The listing builds one solid part. Answer for the finished solid, in the listing's coordinates (mm). Coordinates: 2 decimals unless noted, no trailing zeros. Order: outer loops, then holes, each group sorted by start corner. A loop starts at its lowest first (then second) coordinate and runs counter-clockwise, first axis right, second up. Notation, with made-up numbers: (77.5, 67) -> (116.5, 67) arc R24 ccw to (116.5, 96) -> close; hole circle Ø8 at (69.5, 78). An arc over 180 degrees is marked (long way). Answer in a Markdown table with one row per item.
```python
from build123d import *

# Parameters (mm, degrees)
BOSS_EXTRUDE1_DEPTH = 17
SKETCH2_R           = 2.5
CUT_EXTRUDE1_DEPTH  = 127.546434165
SKETCH3_R           = 1.7
CUT_EXTRUDE2_DEPTH  = 127.546434165


with BuildPart() as part:
    # Sketch1 → Boss-Extrude1 (new body)
    with BuildSketch(Plane.XY):
        with BuildLine():
            Line((3.328897286, -9.429657621), (-95.00665407, -44.144486432))
            ThreePointArc((-95.00665407, -44.144486432), (-113.476816743, -36.586001098), (-108.091360043, -17.369485653))
            Line((-108.091360043, -17.369485653), (-5.394240028, 48.420342898))
            ThreePointArc((-5.394240028, 48.420342898), (2.050554972, 49.787503477), (8.320502943, 45.547001962))
            Line((8.320502943, 45.547001962), (28.320502943, 15.547001962))
            ThreePointArc((28.320502943, 15.547001962), (29.664996488, 7.433320648), (24.472135955, 1.05572809))
            Line((24.472135955, 1.05572809), (4.472135955, -8.94427191))
            ThreePointArc((4.472135955, -8.94427191), (3.908059586, -9.204730863), (3.328897286, -9.429657621))
        make_face()
    extrude(amount=BOSS_EXTRUDE1_DEPTH)

    # Sketch2 → Cut-Extrude1 (cut, through all)
    with BuildSketch(Plane.XY.offset(17)):
        with Locations((-100, -30)):
            Circle(SKETCH2_R)
        Circle(SKETCH2_R)
        with Locations((0, 40)):
            Circle(SKETCH2_R)
        with Locations((20, 10)):
            Circle(SKETCH2_R)
    extrude(amount=-CUT_EXTRUDE1_DEPTH, mode=Mode.SUBTRACT)

    # Sketch3 → Cut-Extrude2 (cut, through all)
    with BuildSketch(Plane.XY.offset(17)):
        with Locations((-108.5, -30)):
            Circle(SKETCH3_R)
        with Locations((-91.5, -30)):
            Circle(SKETCH3_R)
    extrude(amount=-CUT_EXTRUDE2_DEPTH, mode=Mode.SUBTRACT)


solid = part.part
```
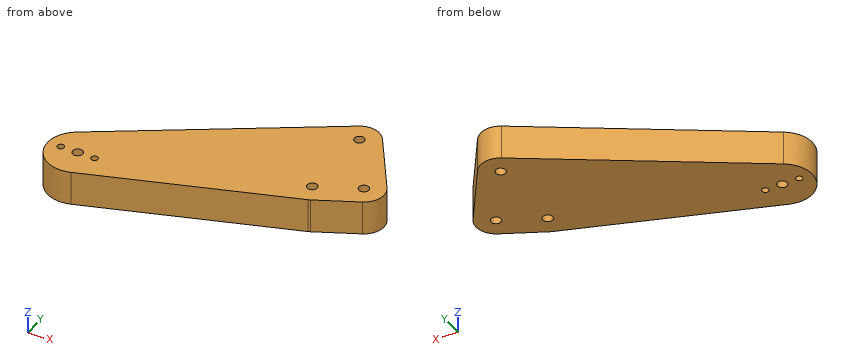
(1) Flat-ended cylindrical pins translate along their axes: pin 1 (1 mm diameter, centred on y = -3.5, z = 12.5, fed in from -X); pin 2 (1 mm diameter, centred on y = 32, z = 14.5, fed in from -X); pin 3 (2 mm diameter, centred on x = 5, z = 10, fed in from +Y). Find the tip coordinate at first contact, or state that the pin passes through.
Check values:
| item | result |
|---|---|
| pin 1 | x = -87.22 |
| pin 2 | x = -31.81 |
| pin 3 | y = 49.17 |
(2) A cutting plane is placed at D-D, the plane y = 40. Determine the outline of the cut face in (x, z), then the cut area to 3 significant figures.
Check values:
| item | result |
|---|---|
| outline | (-18.54, 0) -> (-2.5, 0) -> (-2.5, 17) -> (-18.54, 17) -> close; (2.5, 0) -> (12.02, 0) -> (12.02, 17) -> (2.5, 17) -> close |
| area | 434 mm² |
(3) A cutting plane is placed at A-A, the plane y = -30. Determine the outline of the cut face in (x, z), then the cut area to 3 significant figures.
Check values:
| item | result |
|---|---|
| outline | (-115, 0) -> (-110.2, 0) -> (-110.2, 17) -> (-115, 17) -> close; (-106.8, 0) -> (-102.5, 0) -> (-102.5, 17) -> (-106.8, 17) -> close; (-97.5, 0) -> (-93.2, 0) -> (-93.2, 17) -> (-97.5, 17) -> close; (-89.8, 0) -> (-54.94, 0) -> (-54.94, 17) -> (-89.8, 17) -> close |
| area | 820 mm² |
(4) Find the intervals of material crossed by line 1 along Y through (x, z) = (1, 6.25); line 2 along X through (y, z) = (9, 6); line 3 along Y through (x, z) = (8, 14.75), in increasing order. Write a range as from..to.
Check values:
| item | result |
|---|---|
| line 1 | -10.25..-2.29, 2.29..37.71, 42.29..49.95 |
| line 2 | -66.93..17.71, 22.29..29.95 |
| line 3 | -7.18..46 |
(5) A cutting plane is placed at B-B, the plane z = 5.25. Determine the outline of the cut face in (x, y), then the cut area to 3 significant figures.
Check values:
| item | result |
|---|---|
| outline | (-108.09, -17.37) arc R15 ccw to (-95.01, -44.14) -> (3.33, -9.43) arc R10 ccw to (4.47, -8.94) -> (24.47, 1.06) arc R10 ccw to (28.32, 15.55) -> (8.32, 45.55) arc R10 ccw to (-5.39, 48.42) -> close; hole circle Ø3.4 at (-108.5, -30); hole circle Ø5 at (-100, -30); hole circle Ø3.4 at (-91.5, -30); hole circle Ø5 at (0, 0); hole circle Ø5 at (0, 40); hole circle Ø5 at (20, 10) |
| area | 6,210 mm² |
(6) A cutting plane is placed at C-C, the plane x = -100. Determine the outline of the cut face in (y, z), then the cut area to 3 significant figures.
Check values:
| item | result |
|---|---|
| outline | (-45, 0) -> (-32.5, 0) -> (-32.5, 17) -> (-45, 17) -> close; (-27.5, 0) -> (-12.19, 0) -> (-12.19, 17) -> (-27.5, 17) -> close |
| area | 473 mm² |
